Design review of the part built by this model. Coordinates are the model's own, in mm. Face numbers are marked on the shaded views. A direction names the side the tool comes from. Give positions to 0.01 mm unless a question says otherwise; leave off trailing zeros. Loops run counter-clockwise (first coordinate to the right, second up) from the corner with the lowest first, then second, coordinate; pieces in that order, holes last. Notation, with made-up numbers: M 41.25,7 L 46.25,7 A24 cw 46.25,34 Z; hole C 81.5,40.5 d8. An arc over 180 degrees is marked long. Use a Markdown table: item, result. Add a question column.
(1) Add section B-B, the plane x = -23.5. Give the boundary of the cut face in (y, z), then the cut area to 3 significant figures.
(2) For probe 1 along X at (y, z) = (0.2, 18.5); probe 2 along X at (y, z) = (1.25, 17); probe 3 along Y at (x, z) = (-11, 4), list the stretches that pass through material, from the lowest coordinate up.
(3) Add section C-C, the plane z = -8.5. Give the boundary of the cut face in (x, y), then the cut area to 3 significant figures.
(4) Add section D-D, the plane x = -30.5. Give the boundary of the cut face in (y, z).
(5) Insertion check: pin 1 Ø4 at (x, z) = (-12, -11.5) entering from +Y; pin 2 Ø0.9 at (x, y) = (-9, 2) entering from -Z; pin 3 Ø5 at (x, z) = (12.5, 18) entering from +Y; pin 4 Ø10 at (x, z) = (6, -17.5) entering from -Y. Each pin has a flat end and moves straight along its axis. Give the tip position at first contact, or say it passes through.
(6) Add section A-A, the plane y = 2.5. Give the boundary of the cut face in (x, z).
(7) For the marked faces 1, 2, 3 and 4, list the 3-axis set-ups (+Z, -Z, +X, -X, +Y, -Y) from which the entire face can be reached by the end or side of a thin tool; tool diameter is ignored.
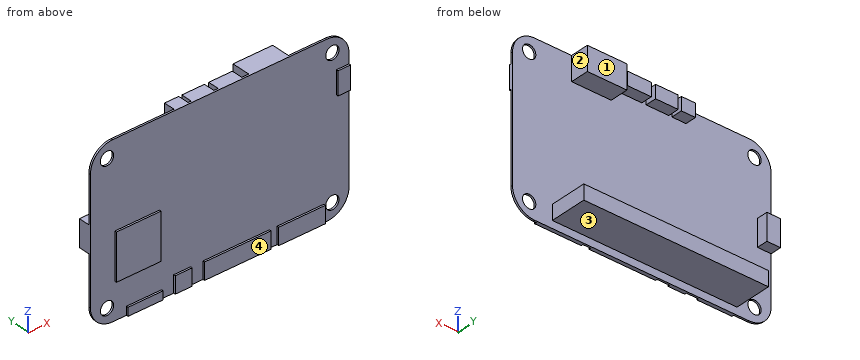
```python
from build123d import *

# Parameters (mm, degrees)
SKETCH_1_W          = 70
SKETCH_1_H          = 45
EXTRUDE_1_DEPTH     = 0.5
FILLET_1_R          = 6
SKETCH_3_R          = 1.8
CUT_EXTRUDE_1_DEPTH = 1
SKETCH_4_W          = 50
SKETCH_4_H          = 4
EXTRUDE_2_DEPTH     = 10
SKETCH_5_W          = 9.523878632
SKETCH_5_H          = 2.249484867
SKETCH_5_W_2        = 4.565570684
SKETCH_5_H_2        = 4.556816288
SKETCH_5_W_3        = 17.967729791
SKETCH_5_W_4        = 12.616684579
SKETCH_5_W_5        = 12.076670843
SKETCH_5_H_3        = 12.420315948
SKETCH_5_W_6        = 3.409196393
SKETCH_5_H_4        = 6.234704053
EXTRUDE_3_DEPTH     = 0.5
SKETCH_6_W          = 10.728619563
SKETCH_6_H          = 6.475095536
EXTRUDE_4_DEPTH     = 5
SKETCH_7_W          = 6.406526606
SKETCH_7_H          = 3.574973131
SKETCH_7_W_2        = 6.136519737
SKETCH_7_W_3        = 3.829188316
SKETCH_7_W_4        = 3.70374934
SKETCH_7_H_2        = 7.167455053
EXTRUDE_5_DEPTH     = 3


with BuildPart() as part:
    # 草图1 → 凸台-拉伸1 (new body)
    with BuildSketch(Plane(origin=(0, 0, 0), x_dir=(1, 0, 0), z_dir=(0, 1, 0))):
        Rectangle(SKETCH_1_W, SKETCH_1_H)
    extrude(amount=EXTRUDE_1_DEPTH)

    # 圆角1
    fillet_1_edges = [part.edges().sort_by_distance(p)[0] for p in [
        (-35, 0.25, -22.5),
        (35, 0.25, -22.5),
        (35, 0.25, 22.5),
        (-35, 0.25, 22.5),
    ]]
    fillet(fillet_1_edges, radius=FILLET_1_R)

    # 草图3 → 切除-拉伸1 (cut)
    with BuildSketch(Plane(origin=(0, 0.5, 0), x_dir=(1, 0, 0), z_dir=(0, 1, 0))):
        with Locations(Location((30.5, 18.5, 0), (0, 0, 270))):
            Circle(SKETCH_3_R)
        with Locations(Location((30.5, -18.5, 0), (0, 0, 270))):
            Circle(SKETCH_3_R)
        with Locations(Location((-30.5, -18.5, 0), (0, 0, 270))):
            Circle(SKETCH_3_R)
        with Locations(Location((-30.5, 18.5, 0), (0, 0, 270))):
            Circle(SKETCH_3_R)
    extrude(amount=-CUT_EXTRUDE_1_DEPTH, mode=Mode.SUBTRACT)

    # 草图4 → 凸台-拉伸2 (add)
    with BuildSketch(Plane(origin=(0, 0.5, 0), x_dir=(1, 0, 0), z_dir=(0, 1, 0))):
        with Locations((-0.770536001, 18.5)):
            Rectangle(SKETCH_4_W, SKETCH_4_H)
    extrude(amount=EXTRUDE_2_DEPTH)

    # 草图5 → 凸台-拉伸3 (add)
    with BuildSketch(Plane.XZ):
        with Locations((-20.495975922, -21.375257567)):
            Rectangle(SKETCH_5_W, SKETCH_5_H)
        with Locations((-10.162076685, -20.221591856)):
            Rectangle(SKETCH_5_W_2, SKETCH_5_H_2)
        with Locations((4.491932447, -20.221591856)):
            Rectangle(SKETCH_5_W_3, SKETCH_5_H_2)
        with Locations((21.846010265, -20.221591856)):
            Rectangle(SKETCH_5_W_4, SKETCH_5_H_2)
        with Locations((-22.361477923, -6.529257)):
            Rectangle(SKETCH_5_W_5, SKETCH_5_H_3)
        with Locations((33.295401803, 10.702090421)):
            Rectangle(SKETCH_5_W_6, SKETCH_5_H_4)
    extrude(amount=EXTRUDE_3_DEPTH)

    # 草图6 → 凸台-拉伸4 (add)
    with BuildSketch(Plane(origin=(0, 0.5, 0), x_dir=(1, 0, 0), z_dir=(0, 1, 0))):
        with Locations((13.653186787, -19.262452232)):
            Rectangle(SKETCH_6_W, SKETCH_6_H)
    extrude(amount=EXTRUDE_4_DEPTH)

    # 草图7 → 凸台-拉伸5 (add)
    with BuildSketch(Plane(origin=(0, 0.5, 0), x_dir=(1, 0, 0), z_dir=(0, 1, 0))):
        with Locations((3.203263303, -20.712513434)):
            Rectangle(SKETCH_7_W, SKETCH_7_H)
        with Locations((-4.22192558, -20.712513434)):
            Rectangle(SKETCH_7_W_2, SKETCH_7_H)
        with Locations((-10.03934629, -20.712513434)):
            Rectangle(SKETCH_7_W_3, SKETCH_7_H)
        with Locations((-33.14812533, -0.22091471)):
            Rectangle(SKETCH_7_W_4, SKETCH_7_H_2)
    extrude(amount=EXTRUDE_5_DEPTH)


solid = part.part
```
Established:
| question | item | result |
|---|---|---|
| 1 | outline | M -0.5,-22.5 L 0.5,-22.5 L 0.5,-20.5 L 10.5,-20.5 L 10.5,-16.5 L 0.5,-16.5 L 0.5,22.5 L 0,22.5 L 0,-0.32 L -0.5,-0.32 L -0.5,-12.74 L 0,-12.74 L 0,-20.25 L -0.5,-20.25 Z |
| 1 | area | 69.8 mm^2 |
| 2 | probe 1 | -34.66 to -32.3, -28.7 to 28.7, 32.3 to 34.66 |
| 2 | probe 2 | 8.29 to 19.02 |
| 2 | probe 3 | 0 to 0.5 |
| 3 | outline | M -35,0 L -28.4,0 L -28.4,-0.5 L -16.32,-0.5 L -16.32,0 L 35,0 L 35,0.5 L -35,0.5 Z |
| 3 | area | 41.0 mm^2 |
| 4 | outline | M 0,-22.31 L 0.5,-22.31 L 0.5,-20.3 L 0,-20.3 Z; M 0,-16.7 L 0.5,-16.7 L 0.5,16.7 L 0,16.7 Z; M 0,20.3 L 0.5,20.3 L 0.5,22.31 L 0,22.31 Z |
| 5 | pin 1 | y = 0.5 |
| 5 | pin 2 | z = -20.5 |
| 5 | pin 3 | y = 5.5 |
| 5 | pin 4 | y = -0.5 |
| 6 | outline | M -35,-3.36 L -31.3,-3.36 L -31.3,3.8 L -35,3.8 Z; M -25.77,-20.5 L 24.23,-20.5 L 24.23,-16.5 L -25.77,-16.5 Z; M -11.95,18.93 L -8.12,18.93 L -8.12,22.5 L -11.95,22.5 Z; M -7.29,18.93 L -1.15,18.93 L -1.15,22.5 L -7.29,22.5 Z; M 0,18.93 L 6.41,18.93 L 6.41,22.5 L 0,22.5 Z; M 8.29,16.02 L 19.02,16.02 L 19.02,22.5 L 8.29,22.5 Z |
| 7 | face 1 | +Z, +X, -X, +Y |
| 7 | face 2 | +Z, +X, +Y |
| 7 | face 3 | -Z, +X, -X, +Y |
| 7 | face 4 | +Z, -Z, +X, -X, -Y |
